Job drawing, mm, ordinate dimensions from the low corner. One solid piece. Coordinates: 2 decimals unless noted, no trailing zeros. Write each loop counter-clockwise with the first axis right and the second up, starting at its lowest first coordinate (ties: lowest second). Pieces come first, ordered by that corner, then holes. Notation, with made-up numbers: (41.5, 11.5) - (54.5, 11.5) arc R21 cw to (54.5, 27.5) - close; hole circle Ø7 at (-36, 53). An arc over 180 degrees is marked (long way). Put each result on its own line as item: value. Start each with the question number.
1. Drop flat-ended pins along their axis: P1, Ø15, axis at y = 24, z = 124, coming from the -X side; P2, Ø6, axis at x = 12, z = 148.5, coming from the +Y side; P3, Ø2.5, axis at x = 20.5, z = 175, coming from the +Y side; P4, Ø9, axis at x = 20.5, y = 33.5, coming from the +Z side. Give the stop position or say it passes through.
2. Saw through at D-D, the plane x = 10.5. Write the cut outline in (y, z), plus the area to 3 significant figures.
3. Saw through at C-C, the plane x = 20.5. Write the cut outline in (y, z).
4. Saw through at A-A, the plane y = 18. Write the cut outline in (x, z).
5. Saw through at B-B, the plane z = 3.5. Write the cut outline in (x, y).
6. Drill centre lines: L1, parallel to X at y = 14.5, z = 143; L2, parallel to Z at x = 22.25, y = 3.5; L3, parallel to Y at x = 1.5, z = 198.5. Where is each one in solid material? Low to high. Write a range as from..to.
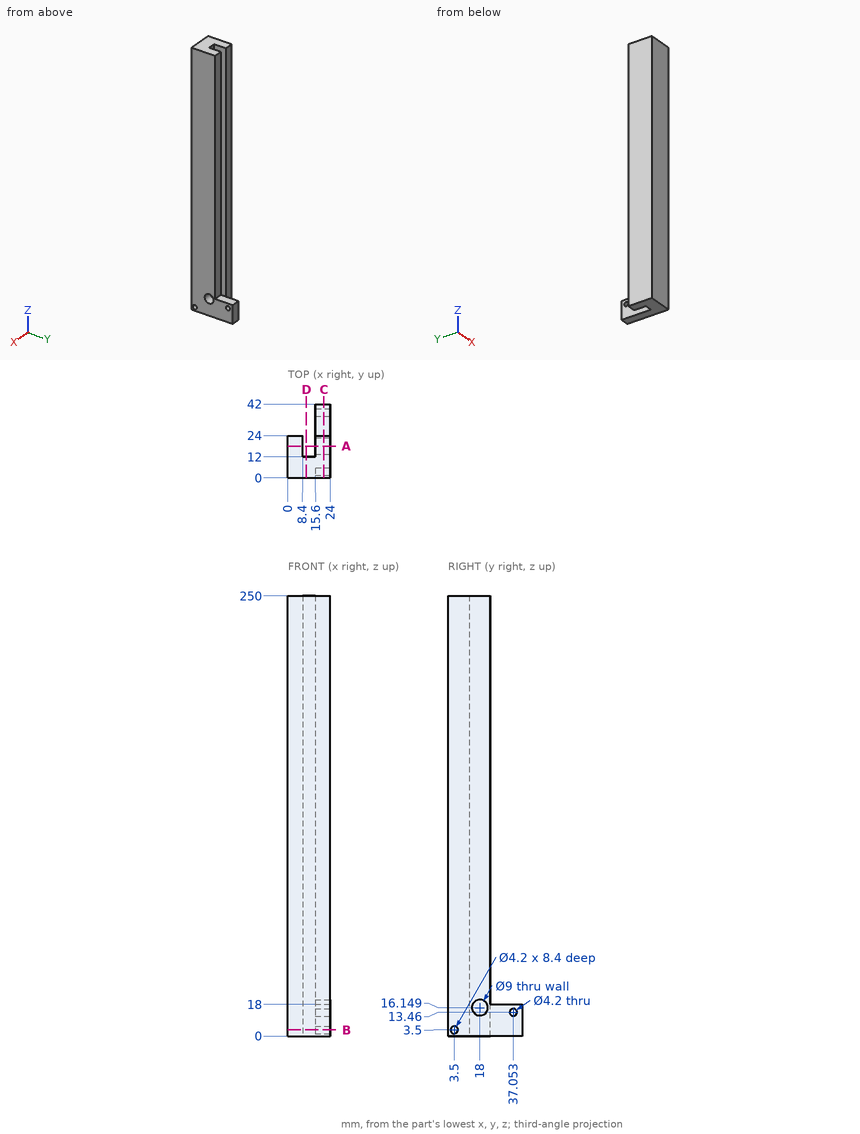
Final values:
1. P1: stops at x = 0
1. P2: stops at y = 12
1. P3: stops at y = 24
1. P4: stops at z = 18
2. outline: (0, 0) - (12, 0) - (12, 250) - (0, 250) - close
2. area: 3,000 mm²
3. outline: (0, 0) - (42, 0) - (42, 18) - (24, 18) - (24, 250) - (0, 250) - close; hole circle Ø4.2 at (3.5, 3.5); hole circle Ø9 at (18, 16.15); hole circle Ø4.2 at (37.05, 13.46)
4. outline: (0, 0) - (8.4, 0) - (8.4, 250) - (0, 250) - close; (15.6, 0) - (24, 0) - (24, 11.65) - (15.6, 11.65) - close; (15.6, 20.65) - (24, 20.65) - (24, 250) - (15.6, 250) - close
5. outline: (0, 0) - (24, 0) - (24, 1.4) - (15.6, 1.4) - (15.6, 5.6) - (24, 5.6) - (24, 42) - (15.6, 42) - (15.6, 12) - (8.4, 12) - (8.4, 24) - (0, 24) - close
6. L1: x = 0..8.4, 15.6..24
6. L2: z = 0..1.4, 5.6..250
6. L3: y = 0..24
